from build123d import *

# Parameters (mm, degrees)
SKETCH_1_R               = 1.6
EXTRUDE_1_DEPTH          = 3
SKETCH_2_R               = 1.6
CUT_EXTRUDE_1_DEPTH      = 85.055041491
SKETCH_3_R               = 1.6
CUT_EXTRUDE_2_DEPTH      = 85.055041491
CUT_EXTRUDE_3_DEPTH      = 85.055041491
CUT_EXTRUDE_3_DEPTH_BACK = 85.055041491


with BuildPart() as part:
    # 草图1 → 凸台-拉伸1 (new body)
    with BuildSketch(Plane(origin=(0, 0, 0), x_dir=(1, 0, 0), z_dir=(0, 1, 0))):
        with BuildLine():
            Line((-62.5, 50), (62.5, 50))
            ThreePointArc((62.5, 50), (66.035533906, 48.535533906), (67.5, 45))
            Line((67.5, 45), (67.5, -45))
            ThreePointArc((67.5, -45), (66.035533906, -48.535533906), (62.5, -50))
            Line((62.5, -50), (-62.5, -50))
            ThreePointArc((-62.5, -50), (-66.035533906, -48.535533906), (-67.5, -45))
            Line((-67.5, -45), (-67.5, 45))
            ThreePointArc((-67.5, 45), (-66.035533906, 48.535533906), (-62.5, 50))
        make_face()
        with Locations(Location((-62.5, 45, 0), (0, 0, 270))):
            Circle(SKETCH_1_R, mode=Mode.SUBTRACT)
        with Locations(Location((62.5, 45, 0), (0, 0, 270))):
            Circle(SKETCH_1_R, mode=Mode.SUBTRACT)
        with Locations(Location((-62.5, -45, 0), (0, 0, 270))):
            Circle(SKETCH_1_R, mode=Mode.SUBTRACT)
        with Locations(Location((62.5, -45, 0), (0, 0, 270))):
            Circle(SKETCH_1_R, mode=Mode.SUBTRACT)
    extrude(amount=EXTRUDE_1_DEPTH)

    # 草图2 → 切除-拉伸1 (cut, through all)
    with BuildSketch(Plane(origin=(0, 3, 0), x_dir=(1, 0, 0), z_dir=(0, 1, 0))):
        with Locations(Location((-24.625, -41.5, 0), (0, 0, 270))):
            Circle(SKETCH_2_R)
        with Locations(Location((-24.625, -21.5, 0), (0, 0, 270))):
            Circle(SKETCH_2_R)
        with Locations(Location((-1.875, -41.5, 0), (0, 0, 270))):
            Circle(SKETCH_2_R)
        with Locations(Location((-1.875, -21.5, 0), (0, 0, 270))):
            Circle(SKETCH_2_R)
        with Locations(Location((24.75, -41.5, 0), (0, 0, 270))):
            Circle(SKETCH_2_R)
        with Locations(Location((24.75, -21.5, 0), (0, 0, 270))):
            Circle(SKETCH_2_R)
    extrude(amount=-CUT_EXTRUDE_1_DEPTH, mode=Mode.SUBTRACT)

    # 草图3 → 切除-拉伸2 (cut, through all)
    with BuildSketch(Plane(origin=(0, 3, 0), x_dir=(1, 0, 0), z_dir=(0, 1, 0))):
        with Locations(Location((-27, -36, 0), (0, 0, 270))):
            Circle(SKETCH_3_R)
        with Locations(Location((27, -36, 0), (0, 0, 90))):
            Circle(SKETCH_3_R)
        with Locations(Location((-27, 6.92, 0), (0, 0, 270))):
            Circle(SKETCH_3_R)
        with Locations(Location((27, 6.92, 0), (0, 0, 90))):
            Circle(SKETCH_3_R)
        with Locations(Location((-27, -26, 0), (0, 0, 270))):
            Circle(SKETCH_3_R)
        with Locations(Location((27, -26, 0), (0, 0, 90))):
            Circle(SKETCH_3_R)
    extrude(amount=-CUT_EXTRUDE_2_DEPTH, mode=Mode.SUBTRACT)

    # 草图6 → 切除-拉伸3 (cut, two sides: drawn at the far end of the back side and taken through both)
    with BuildSketch(Plane(origin=(0, 3, 0), x_dir=(1, 0, 0), z_dir=(0, 1, 0)).offset(-CUT_EXTRUDE_3_DEPTH_BACK)):
        with BuildLine():
            ThreePointArc((-54.5, 10.92), (-56.621320344, 11.798679656), (-57.5, 13.92))
            Line((-57.5, 13.92), (-57.5, 34))
            ThreePointArc((-57.5, 34), (-55.742640687, 38.242640687), (-51.5, 40))
            Line((-51.5, 40), (-34, 40))
            ThreePointArc((-34, 40), (-31.878679656, 39.121320344), (-31, 37))
            Line((-31, 37), (-31, 13.92))
            ThreePointArc((-31, 13.92), (-31.878679656, 11.798679656), (-34, 10.92))
            Line((-34, 10.92), (-54.5, 10.92))
        make_face()
        with BuildLine():
            ThreePointArc((-20, 10.92), (-22.121320344, 11.798679656), (-23, 13.92))
            Line((-23, 13.92), (-23, 37))
            ThreePointArc((-23, 37), (-22.121320344, 39.121320344), (-20, 40))
            Line((-20, 40), (20, 40))
            ThreePointArc((20, 40), (22.121320344, 39.121320344), (23, 37))
            Line((23, 37), (23, 13.92))
            ThreePointArc((23, 13.92), (22.121320344, 11.798679656), (20, 10.92))
            Line((20, 10.92), (-20, 10.92))
        make_face()
        with BuildLine():
            ThreePointArc((31, 37), (31.878679656, 39.121320344), (34, 40))
            Line((34, 40), (51.5, 40))
            ThreePointArc((51.5, 40), (55.742640687, 38.242640687), (57.5, 34))
            Line((57.5, 34), (57.5, 13.92))
            ThreePointArc((57.5, 13.92), (56.621320344, 11.798679656), (54.5, 10.92))
            Line((54.5, 10.92), (34, 10.92))
            ThreePointArc((34, 10.92), (31.878679656, 11.798679656), (31, 13.92))
            Line((31, 13.92), (31, 37))
        make_face()
        with BuildLine():
            Line((57.5, -11), (57.5, -0.08))
            ThreePointArc((57.5, -0.08), (56.621320344, 2.041320344), (54.5, 2.92))
            Line((54.5, 2.92), (34, 2.92))
            ThreePointArc((34, 2.92), (31.878679656, 2.041320344), (31, -0.08))
            Line((31, -0.08), (31, -10))
            ThreePointArc((31, -10), (31.878679656, -12.121320344), (34, -13))
            Line((34, -13), (40, -13))
            Line((40, -13), (40, -14))
            Line((40, -14), (54.5, -14))
            ThreePointArc((54.5, -14), (56.621320344, -13.121320344), (57.5, -11))
        make_face()
        with BuildLine():
            ThreePointArc((-23, -0.08), (-22.121320344, 2.041320344), (-20, 2.92))
            Line((-20, 2.92), (20, 2.92))
            ThreePointArc((20, 2.92), (22.121320344, 2.041320344), (23, -0.08))
            Line((23, -0.08), (23, -10))
            ThreePointArc((23, -10), (22.121320344, -12.121320344), (20, -13))
            Line((20, -13), (-20, -13))
            ThreePointArc((-20, -13), (-22.121320344, -12.121320344), (-23, -10))
            Line((-23, -10), (-23, -0.08))
        make_face()
        with BuildLine():
            Line((-31, -0.08), (-31, -10))
            ThreePointArc((-31, -10), (-31.878679656, -12.121320344), (-34, -13))
            Line((-34, -13), (-40, -13))
            Line((-40, -13), (-40, -14))
            Line((-40, -14), (-54.5, -14))
            ThreePointArc((-54.5, -14), (-56.621320344, -13.121320344), (-57.5, -11))
            Line((-57.5, -11), (-57.5, -0.08))
            ThreePointArc((-57.5, -0.08), (-56.621320344, 2.041320344), (-54.5, 2.92))
            Line((-54.5, 2.92), (-34, 2.92))
            ThreePointArc((-34, 2.92), (-31.878679656, 2.041320344), (-31, -0.08))
        make_face()
        with BuildLine():
            ThreePointArc((-54.5, -22), (-56.621320344, -22.878679656), (-57.5, -25))
            Line((-57.5, -25), (-57.5, -34))
            ThreePointArc((-57.5, -34), (-55.742640687, -38.242640687), (-51.5, -40))
            Line((-51.5, -40), (-43, -40))
            ThreePointArc((-43, -40), (-40.878679656, -39.121320344), (-40, -37))
            Line((-40, -37), (-40, -30.568485257))
            Line((-40, -30.568485257), (-40, -25))
            ThreePointArc((-40, -25), (-40.878679656, -22.878679656), (-43, -22))
            Line((-43, -22), (-54.5, -22))
        make_face()
        with BuildLine():
            Line((57.5, -34), (57.5, -25))
            ThreePointArc((57.5, -25), (56.621320344, -22.878679656), (54.5, -22))
            Line((54.5, -22), (43, -22))
            ThreePointArc((43, -22), (40.878679656, -22.878679656), (40, -25))
            Line((40, -25), (40, -37))
            ThreePointArc((40, -37), (40.878679656, -39.121320344), (43, -40))
            Line((43, -40), (51.5, -40))
            ThreePointArc((51.5, -40), (55.742640687, -38.242640687), (57.5, -34))
        make_face()
    extrude(amount=CUT_EXTRUDE_3_DEPTH + CUT_EXTRUDE_3_DEPTH_BACK, mode=Mode.SUBTRACT)


solid = part.part
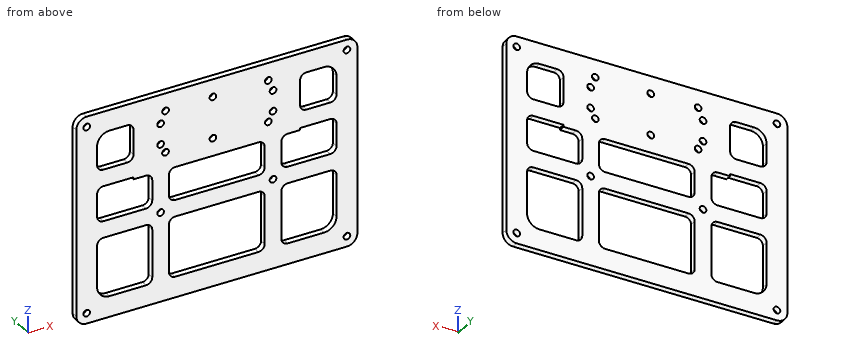
Design review of the part built by this model. Coordinates are the model's own, in mm. Coordinates: 2 decimals unless noted, no trailing zeros. Loops run counter-clockwise (first coordinate to the right, second up) from the corner with the lowest first, then second, coordinate; pieces in that order, holes last. Notation, with made-up numbers: M -21.5,-23.75 L 2.5,-23.75 A33 ccw 2.5,4.25 Z; hole C 3,15.25 d6. An arc over 180 degrees is marked long. Use one line per item in the form item = value.
(1) Consider section C-C (z = 30). Write out the cut boundary in (x, y), and give its area (3 significant figures).
Return value:
outline = M -67.5,0 L -57.5,0 L -57.5,3 L -67.5,3 Z; M -40,0 L 40,0 L 40,3 L -40,3 Z; M 57.5,0 L 67.5,0 L 67.5,3 L 57.5,3 Z
area = 300 mm2
(2) For line 1 along Z through (x, y) = (-37, 1); line 2 along X through (y, z) = (1.95, 32.5); line 3 along X through (y, z) = (1, -45), list the stretches that pass through material, from the lowest coordinate up. Write a range as from..to.
Return value:
line_1 = -50..-40, -10.92..-2.92, 13..50
line_2 = -67.5..-57.5, -40..40, 57.5..67.5
line_3 = -67.5..-64.1, -60.9..60.9, 64.1..67.5
(3) Consider section D-D (y = 2.5). Give the number of separate pieces and of enclosed holes in the cut face, and give its area (3 significant figures).
Return value:
separate_pieces = 1
enclosed_holes = 24
area = 8,310 mm2
(4) Consider section A-A (z = 6.5). Write out the cut boundary in (x, y), and give its area (3 significant figures).
Return value:
outline = M -67.5,0 L -57.5,0 L -57.5,3 L -67.5,3 Z; M -31,0 L -23,0 L -23,3 L -31,3 Z; M 23,0 L 31,0 L 31,3 L 23,3 Z; M 57.5,0 L 67.5,0 L 67.5,3 L 57.5,3 Z
area = 108 mm2
(5) Consider section B-B (x = -32.5). Write out the cut boundary in (y, z), and give its area (3 significant figures).
Return value:
outline = M 0,-50 L 3,-50 L 3,-39.6 L 0,-39.6 Z; M 0,-11.32 L 3,-11.32 L 3,-2.52 L 0,-2.52 Z; M 0,12.6 L 3,12.6 L 3,50 L 0,50 Z
area = 170 mm2
